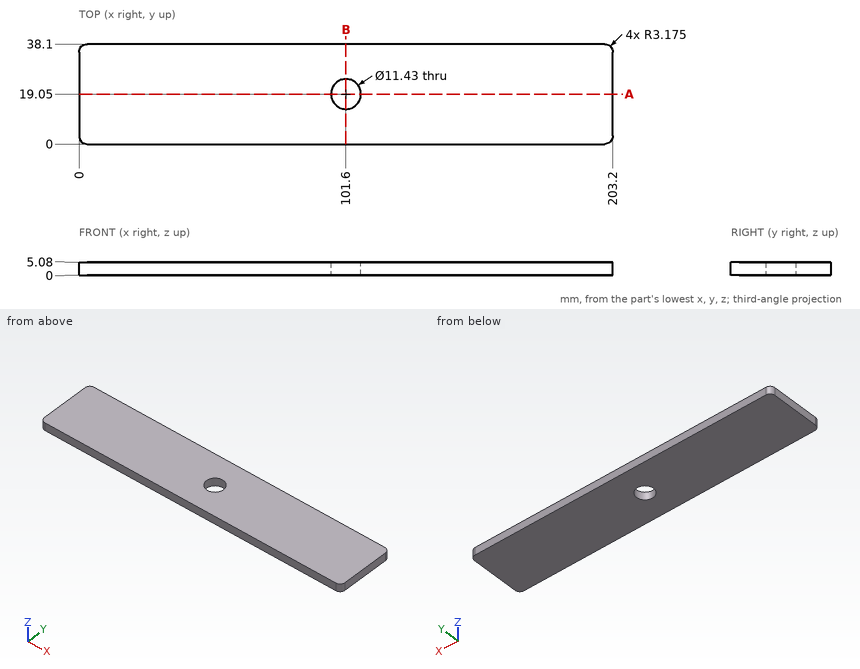
Geometry check sheet. Reference: drawing and pictorial views, mm from the part's lowest x, y, z. Give positions to 0.01 mm unless a question says otherwise; leave off trailing zeros. Write each loop counter-clockwise with the first axis right and the second up, starting at its lowest first coordinate (ties: lowest second). Pieces come first, ordered by that corner, then holes. Notation, with made-up numbers: M 15.5,-20.5 L 53.5,-20.5 A23 ccw 53.5,-6.5 Z; hole C 50.25,-22 d4. An arc over 180 degrees is marked long. Use CSV: the item, a comma, the result in double quotes.
1) Material ranges on line 1 along Y through (x, z) = (102, 4.4); line 2 along X through (y, z) = (14, 1.85); line 3 along X through (y, z) = (22, 0.65), recorded low to high.
Final values:
line 1,"0 to 13.35, 24.75 to 38.1"
line 2,"0 to 98.92, 104.28 to 203.2"
line 3,"0 to 96.71, 106.49 to 203.2"
2) Cross-section at A-A (y = 19.05). Enter the section's corners in (x, z) (3 decimals).
Final values:
outline,"M 0,0 L 95.885,0 L 95.885,5.08 L 0,5.08 Z; M 107.315,0 L 203.2,0 L 203.2,5.08 L 107.315,5.08 Z"
3) Cross-section at B-B (x = 101.6). Enter the section's corners in (y, z) (3 decimals).
Final values:
outline,"M 0,0 L 13.335,0 L 13.335,5.08 L 0,5.08 Z; M 24.765,0 L 38.1,0 L 38.1,5.08 L 24.765,5.08 Z"
4) Go/stop test with a flat-tipped pin: pin 1 Ø4 at (x, y) = (26, 18) entering from -Z. Record where the tip stops, or that it passes through.
Final values:
pin 1,"z = 0"
